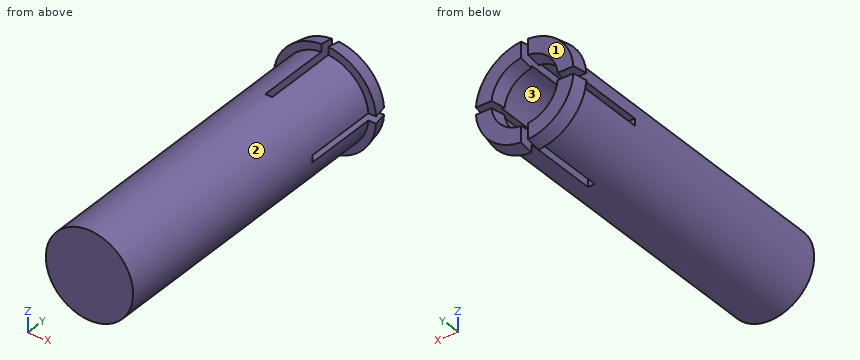
```python
from build123d import *

# Parameters (mm, degrees)
F0_R     = 12.5
F0_R_2   = 9.525
F1_DEPTH = 81.026
F2_R     = 14
F2_R_2   = 9.525
F3_DEPTH = 4
F3_TAPER = -10
F4_W     = 16.5
F4_H     = 2
F4_W_2   = 2
F4_H_2   = 16.5
F5_DEPTH = 25.4
F6_R     = 12.5
F7_DEPTH = 12.7


with BuildPart() as f1:
    # F0 (on Front) → F1 (new body)
    with BuildSketch(Plane.XZ):
        Circle(F0_R)
        Circle(F0_R_2, mode=Mode.SUBTRACT)
    extrude(amount=F1_DEPTH)

    # F2 (on face) → F3 (join)
    with BuildSketch(Plane(origin=(0, 0, 0), x_dir=(-1, 0, 0), z_dir=(0, 1, 0))):
        Circle(F2_R)
        Circle(F2_R_2, mode=Mode.SUBTRACT)
    extrude(amount=-F3_DEPTH, taper=F3_TAPER)

    # F4 (on face) → F5 (cut)
    with BuildSketch(Plane.XZ):
        with Locations((-9.25, 0)):
            Rectangle(F4_W, F4_H)
        with Locations((0, 9.25)):
            Rectangle(F4_W_2, F4_H_2)
        Rectangle(F4_W_2, F4_H)
        with Locations((9.25, 0)):
            Rectangle(F4_W, F4_H)
        with Locations((0, -9.25)):
            Rectangle(F4_W_2, F4_H_2)
    extrude(amount=F5_DEPTH, mode=Mode.SUBTRACT)

    # F6 (on face) → F7 (join)
    with BuildSketch(Plane.XZ.offset(81.026)):
        Circle(F6_R)
    extrude(amount=F7_DEPTH)


solid = f1.part
```
Part model, mm, in its own coordinate system. Face numbers are marked on the shaded views. Round coordinates to 2 decimals unless told otherwise and drop trailing zeros. Write each loop counter-clockwise with the first axis right and the second up, starting at its lowest first coordinate (ties: lowest second). Pieces come first, ordered by that corner, then holes. Notation, with made-up numbers: M 15,11 L 62,11 A16 cw 62,38 Z; hole C 58.25,-0.5 d8. An arc over 180 degrees is marked long. One line per question, with ' | ' between items.
(1) Saw through at C-C on y = -22.5. Write the cut outline in (x, z) (3 decimals), then the cut area to 3 significant figures.
Answer key:
outline: M -12.46,-1 A12.5 ccw -1,-12.46 L -1,-9.472 A9.525 cw -9.472,-1 Z; M -12.46,1 L -9.472,1 A9.525 cw -1,9.472 L -1,12.46 A12.5 ccw Z; M 1,-12.46 A12.5 ccw 12.46,-1 L 9.472,-1 A9.525 cw 1,-9.472 Z; M 1,9.472 A9.525 cw 9.472,1 L 12.46,1 A12.5 ccw 1,12.46 Z | area: 182 mm^2
(2) Saw through at B-B on z = 0. Write the cut outline in (x, y) (3 decimals).
Answer key:
outline: M -12.5,-93.726 L 12.5,-93.726 L 12.5,-25.4 L 9.525,-25.4 L 9.525,-81.026 L -9.525,-81.026 L -9.525,-25.4 L -12.5,-25.4 Z
(3) Pin check, flat tips, straight feed: pin 1 (3 mm diameter, centred on y = -12.5, z = 10.5, fed in from +X); pin 2 (4 mm diameter, centred on x = 9.5, z = -10, fed in from -Y); pin 3 (1 mm diameter, centred on x = 0, z = 11.5, fed in from +Y); pin 4 (5 mm diameter, centred on y = -59.5, z = -5, fed in from +X). Stop position of each tip, or through.
Answer key:
pin 1: stops at x = 8.67 | pin 2: stops at y = -93.73 | pin 3: stops at y = -25.4 | pin 4: stops at x = 12.25
(4) Two-plate mould, pull along Y, no slides. Class the marked faces 1, 2 and 3: released by +Y, released by -Y, zero draft, split by the parting line, or undercut.
Answer key:
face 1: released by +Y | face 2: zero draft | face 3: undercut
(5) Saw through at A-A on x = 0. Write the cut outline in (y, z) (3 decimals).
Answer key:
outline: M -93.726,-12.5 L -25.4,-12.5 L -25.4,-9.525 L -81.026,-9.525 L -81.026,9.525 L -25.4,9.525 L -25.4,12.5 L -93.726,12.5 Z
(6) Probe line 1 along Z through (x, y) = (0, -42.5) (3 decimals); line 2 along Z through (x, y) = (-7.75, -6.5). List the from-to ranges inside material, lowest first.
Answer key:
line 1: z = -12.5 to -9.525, 9.525 to 12.5 | line 2: z = -9.81 to -5.54, 5.54 to 9.81
